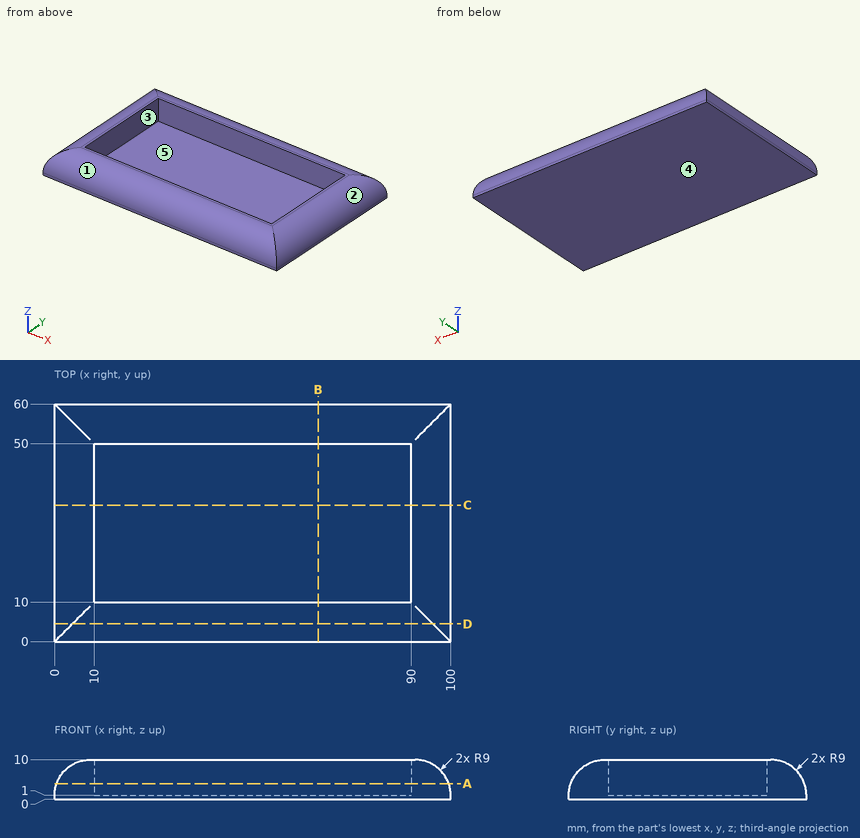
Verification items for this drawing (mm, ordinates from the low corner). A direction names the side the tool comes from. Round coordinates to 2 decimals unless told otherwise and drop trailing zeros. Write each loop counter-clockwise with the first axis right and the second up, starting at its lowest first coordinate (ties: lowest second). Pieces come first, ordered by that corner, then holes. Notation, with made-up numbers: (72, 74.5) - (131, 74.5) arc R20 cw to (131, 90.5) - close; hole circle Ø5 at (36, 71.5). An arc over 180 degrees is marked (long way). Answer as a JSON object with one key per item and string values. Group by question number.
Q1. Section check B-B, the plane x = 66.5. Enter the section's corners in (y, z).
Q2. Go/stop test with flat-tipped pins: pin 1 Ø12 at (x, y) = (67, 35) entering from +Z; pin 2 Ø6 at (y, z) = (47, 6.5) entering from -X; pin 3 Ø2.5 at (x, z) = (40.5, 3.5) entering from +Y; pin 4 Ø1.5 at (x, y) = (69.5, 10.5) entering from +Z. Record where each tip stops, or that it passes through.
Q3. Mould release check, pull along X, two halves, no side actions. Record for the marked faces 1, 2 and 3: released by +X, released by -X, zero draft, split by the parting line, or undercut.
Q4. Section check C-C, the plane y = 34.5. Enter the section's corners in (x, z).
Q5. Tool access check on the marked faces 4 and 5. Record the directions out of +Z, -Z, +X, -X, +Y, -Y that give a thin tool (end or side, any length) a straight path to the whole face; none if there is none.
Q6. Section check A-A, the plane z = 4. Enter the section's corners in (x, y), plus the area to 3 significant figures.
Q7. Thickness scan on line 1 (X direction, y = 29, z = 8.5); line 2 (Y direction, x = 49, z = 5.75); line 3 (Z direction, x = 64, y = 20). Record the ranges inside material, lowest first.
Q8. Section check D-D, the plane y = 4.5. Enter the section's corners in (x, z), plus the area to 3 significant figures.
Found:
{
 "1": {"outline": "(0, 0) - (60, 0) - (60, 1) arc R9 ccw to (51, 10) - (50, 10) - (50, 1) - (10, 1) - (10, 10) - (9, 10) arc R9 ccw to (0, 1) - close"},
 "2": {"pin 1": "stops at z = 1", "pin 2": "stops at x = 0.35", "pin 3": "stops at y = 59.91", "pin 4": "stops at z = 10"},
 "3": {"face 1": "zero draft", "face 2": "released by +X", "face 3": "undercut"},
 "4": {"outline": "(0, 0) - (100, 0) - (100, 1) arc R9 ccw to (91, 10) - (90, 10) - (90, 1) - (10, 1) - (10, 10) - (9, 10) arc R9 ccw to (0, 1) - close"},
 "5": {"face 4": "-Z, +X, -X, +Y, -Y", "face 5": "+Z"},
 "6": {"outline": "(0.51, 0.51) - (99.49, 0.51) - (99.49, 59.49) - (0.51, 59.49) - close; hole (10, 10) - (90, 10) - (90, 50) - (10, 50) - close", "area": "2,640 mm^2"},
 "7": {"line 1": "x = 4.03 to 10, 90 to 95.97", "line 2": "y = 1.36 to 10, 50 to 58.64", "line 3": "z = 0 to 1"},
 "8": {"outline": "(0, 0) - (100, 0) - (100, 1) arc R9 ccw to (95.5, 8.79) - (4.5, 8.79) arc R9 ccw to (0, 1) - close", "area": "859 mm^2"}
}
